Verification items for the finished model (mm, model axes). A direction names the side the tool comes from. Give positions to 0.01 mm unless a question says otherwise; leave off trailing zeros. Write each loop counter-clockwise with the first axis right and the second up, starting at its lowest first coordinate (ties: lowest second). Pieces come first, ordered by that corner, then holes. Notation, with made-up numbers: M 9,-5 L 29,-5 A6 ccw 29,3 Z; hole C -15.5,-12.75 d7. An arc over 180 degrees is marked long. Answer as a JSON object with one key per item and string values.
Autodesk Inventor part; units mm, degrees
ref_plane "YZ Plane" through (0, 0, 0) normal (1, 0, 0) x (0, 1, 0)
ref_plane "XZ Plane" through (0, 0, 0) normal (0, 1, 0) x (-1, 0, 0)
ref_plane "XY Plane" through (0, 0, 0) normal (0, 0, 1) x (1, 0, 0)
sketch "Sketch2" plane through (0, 0, 0) normal (0, 0, 1) x (1, 0, 0)
  line L0 (-42.5, 62.5) -> (42.5, 62.5)
  line L1 (42.5, 62.5) -> (42.5, -62.5)
  line L2 (42.5, -62.5) -> (-42.5, -62.5)
  line L3 (-42.5, -62.5) -> (-42.5, 62.5)
  line L4 (-67.5, 92.5) -> (67.5, 92.5)
  line L5 (67.5, 92.5) -> (67.5, -85)
  line L6 (67.5, -85) -> (-67.5, -85)
  line L7 (-67.5, -85) -> (-67.5, 92.5)
  point P0 (0, 0)
  dimension "d16" = 125
  dimension "d17" = 62.5
  dimension "d18" = 85
  dimension "d19" = 42.5
  dimension "d20" = 25
  dimension "d21" = 25
  dimension "d23" = 22.5
  dimension "d75" = 30
extrude "flash4base" add sketch "Sketch2" along normal blind 13.5 contours L0 L1 L2 L3 | L4 L5 L6 L7
sketch "Sketch3" plane through (0, 0, 0) normal (0, 0, -1) x (-1, 0, 0)
  point P0 (0, 0)
  point P1 (-20, 47.65)
  point P2 (20, 47.65)
  point P3 (-20, -47.65)
  point P4 (20, -47.65)
  dimension "d26" = 40
  dimension "d27" = 20
  dimension "d28" = 95.3
  dimension "d29" = 47.65
hole "flash4mountingholes" at (20, 47.65, 0) at (-20, 47.65, 0) at (20, -47.65, 0) at (-20, -47.65, 0) direction (0, 0, 1) diameter 3.4 end through all counterbore diameter 11 counterbore depth 2.6
sketch "Sketch4" plane through (0, 0, 13.5) normal (0, 0, 1) x (1, 0, 0)
  point P0 (0, 0)
  point P1 (50, -50)
  point P2 (-50, -50)
  point P3 (50, 50)
  point P4 (-50, 50)
  dimension "d37" = 100
  dimension "d38" = 50
  dimension "d39" = 100
  dimension "d56" = 50
hole "mountinPostMountingHoles" at (50, -50, 13.5) at (-50, -50, 13.5) at (50, 50, 13.5) at (-50, 50, 13.5) direction (0, 0, -1) diameter 4.5 end through all counterbore diameter 13 counterbore depth 3.4
sketch "Sketch5" plane through (0, 0, 13.5) normal (0, 0, 1) x (1, 0, 0)
  line L0 (-50.3, 30) -> (-48.7, 30)
  line L1 (-46.7, 28) -> (-46.7, -27)
  line L2 (-49.7, -30) -> (-50.3, -30)
  line L3 (-53.3, -27) -> (-53.3, 27)
  line L4 (49.7, 30) -> (50.3, 30)
  line L5 (53.3, 27) -> (53.3, -27)
  line L6 (50.3, -30) -> (49.7, -30)
  line L7 (46.7, -27) -> (46.7, 27)
  arc A0 (-46.7, 28) -> (-48.7, 30) centre (-48.7, 28) ccw
  arc A1 (-50.3, 30) -> (-53.3, 27) centre (-50.3, 27) ccw
  arc A2 (-53.3, -27) -> (-50.3, -30) centre (-50.3, -27) ccw
  arc A3 (-49.7, -30) -> (-46.7, -27) centre (-49.7, -27) ccw
  arc A4 (46.7, -27) -> (49.7, -30) centre (49.7, -27) ccw
  arc A5 (50.3, -30) -> (53.3, -27) centre (50.3, -27) ccw
  arc A6 (49.7, 30) -> (46.7, 27) centre (49.7, 27) ccw
  arc A7 (53.3, 27) -> (50.3, 30) centre (50.3, 27) ccw
  line L8 (-27, 85) -> (27, 85)
  line L9 (30, 82) -> (30, 81.4)
  line L10 (27, 78.4) -> (-27, 78.4)
  line L11 (-30, 81.4) -> (-30, 82)
  line L12 (-27, -65) -> (27, -65)
  line L13 (30, -68) -> (30, -68.6)
  line L14 (27, -71.6) -> (-27, -71.6)
  line L15 (-30, -68.6) -> (-30, -68)
  arc A8 (-27, 85) -> (-30, 82) centre (-27, 82) ccw
  arc A9 (-30, 81.4) -> (-27, 78.4) centre (-27, 81.4) ccw
  arc A10 (30, 82) -> (27, 85) centre (27, 82) ccw
  arc A11 (27, 78.4) -> (30, 81.4) centre (27, 81.4) ccw
  arc A12 (-27, -65) -> (-30, -68) centre (-27, -68) ccw
  arc A13 (-30, -68.6) -> (-27, -71.6) centre (-27, -68.6) ccw
  arc A14 (30, -68) -> (27, -65) centre (27, -68) ccw
  arc A15 (27, -71.6) -> (30, -68.6) centre (27, -68.6) ccw
  point P0 (0, 0)
  point P1 (46.7, 30)
  point P2 (53.3, 30)
  point P3 (-30, -71.6)
  dimension "d48" = 6.6
  dimension "d50" = 6.6
  dimension "d52" = 30
  dimension "d53" = 30
  dimension "d54" = 30
  dimension "d55" = 30
  dimension "d57" = 2
  dimension "d58" = 3
  dimension "d59" = 3
  dimension "d62" = 6.6
  dimension "d63" = 6.6
  dimension "d64" = 30
  dimension "d65" = 30
  dimension "d66" = 30
  dimension "d67" = 30
  dimension "d70" = 3
  dimension "d71" = 93.4
  dimension "d72" = 46.7
  dimension "d73" = 143.4
  dimension "d74" = 65
extrude "m6Alignment" cut sketch "Sketch5" against normal through all
equation "\"d62\" = d50"
equation "\"d63\" = d50"
equation "\"d10\" = 125"
equation "\"d11\" = 7"
equation "\"d12\" = 4"
properties part number "sCMOSmountingBase"
1) Section check A-A on x = 0. Record the boundary of the cut face in (y, z), and give its area (3 significant figures).
Completed:
{"outline": "M -85,0 L -71.6,0 L -71.6,13.5 L -85,13.5 Z; M -65,0 L 78.4,0 L 78.4,13.5 L -65,13.5 Z; M 85,0 L 92.5,0 L 92.5,13.5 L 85,13.5 Z", "area": "2,220 mm2"}
2) Section check C-C on z = 6.5. Count the separate pieces of the cut face and the enclosed holes in it, and give its area (3 significant figures).
Completed:
{"separate pieces": "1", "enclosed holes": "12", "area": "22,300 mm2"}
3) Section check B-B on y = -23. Record the boundary of the cut face in (x, z).
Completed:
{"outline": "M -67.5,0 L -53.3,0 L -53.3,13.5 L -67.5,13.5 Z; M -46.7,0 L 46.7,0 L 46.7,13.5 L -46.7,13.5 Z; M 53.3,0 L 67.5,0 L 67.5,13.5 L 53.3,13.5 Z"}
4) Access from +Z, -Z, +X, -X, +Y, -Y to the whole of each face (thin tool, end or side, straight path). Record for faces 1 (the face through (0, -65, 7)), 2 (the face through (-19, 46, 2.6)), 3 (the face through (-47, 50, 10.1)).
Completed:
{"face 1": "+Z, -Z", "face 2": "-Z", "face 3": "+Z"}
5) Release check for a two-part mould opening along X. For faces 4 (the face through (0, 85, 7)), 5 (the face through (-1, 92.5, 7)), 6 (the face through (67.5, 5, 7)), 7 (the face through (53.3, 0, 7)) record: pulls with the +X half, pulls with the -X half, needs draft (parallel to the pull), parting line crosses it, or undercut.
Completed:
{"face 4": "undercut", "face 5": "needs draft", "face 6": "pulls with the +X half", "face 7": "undercut"}
6) Thickness scan on L1, parallel to Y at x = -20, z = 1.6; L2, parallel to X at y = 17, z = 7.75; L3, parallel to Y at x = -50, z = 7. Record the ranges inside material, lowest first.
Completed:
{"L1": "y = -85 to -71.6, -65 to -53.15, -42.15 to 42.15, 53.15 to 78.4, 85 to 92.5", "L2": "x = -67.5 to -53.3, -46.7 to 46.7, 53.3 to 67.5", "L3": "y = -85 to -52.25, -47.75 to -30, 30 to 47.75, 52.25 to 92.5"}
7) Go/stop test with flat-tipped pins: pin 1 (9 mm diameter, centred on x = -20.5, y = -47, fed in from -Z); pin 2 (11.5 mm diameter, centred on x = 50, y = -50, fed in from +Z). Record where each tip stops, or that it passes through.
Completed:
{"pin 1": "stops at z = 2.6", "pin 2": "stops at z = 10.1"}
